The listing builds one solid part. Answer for the finished solid, in the listing's coordinates (mm). Face numbers are marked on the shaded views. A direction names the side the tool comes from. Coordinates: 2 decimals unless noted, no trailing zeros. Write each loop counter-clockwise with the first axis right and the second up, starting at its lowest first coordinate (ties: lowest second). Pieces come first, ordered by that corner, then holes.
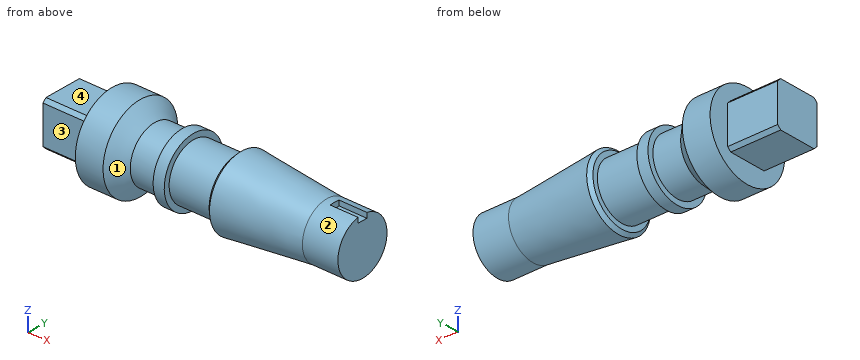
Autodesk Fusion 360 part; units mm, degrees
sketch "Sketch1" plane through (0, 0, 0) normal (0, 1, 0) x (1, 0, 0) in component "Shaft"
  line L0 (0, 0) -> (25, 0)
  line L1 (25, 38) -> (0, 38)
  line L2 (0, 38) -> (0, 0)
  line L3 (25, 38) -> (38, 25)
  line L4 (38, 25) -> (63, 25)
  line L5 (63, 25) -> (63, 30)
  line L6 (63, 30) -> (73, 30)
  line L7 (73, 30) -> (73, 25)
  line L8 (73, 25) -> (113, 25)
  line L9 (113, 25) -> (113, 32.5)
  line L10 (113, 32.5) -> (116, 32.5)
  line L11 (0, 0) -> (193, 0)
  line L12 (116, 32.5) -> (193, 25)
  line L13 (193, 25) -> (225, 25)
  line L14 (225, 25) -> (225, 0)
  line L15 (225, 0) -> (193, 0)
  dimension "d2" = 25
  dimension "d3" = 38
  dimension "d8" = 25
  dimension "d9" = 5
  dimension "d10" = 10
  dimension "d11" = 5
  dimension "d12" = 13
  dimension "d13" = 40
  dimension "d15" = 3
  dimension "d17" = 25
  dimension "d18" = 32
revolve "Revolve1" add sketch "Sketch1" angle 360 about axis through (0, 0, 0) along (1, 0, 0) in component "Shaft"
sketch "Sketch2" plane through (0, 0, 0) normal (-1, 0, 0) x (0, -1, 0) in component "Shaft"
  circle A0 centre (0, 0) radius 38
  line L0 (20, -20) -> (-20, -20)
  line L1 (-20, -20) -> (-20, 20)
  line L2 (-20, 20) -> (20, 20)
  line L3 (20, 20) -> (20, -20)
  line L4 (20, -20) -> (-20, 20) construction
  line L5 (-20, -20) -> (20, 20) construction
  dimension "d20" = 40
  dimension "d21" = 40
extrude "Extrude1" add sketch "Sketch2" along normal blind 45 contours L0 L1 L2 L3 in component "Shaft"
sketch "Sketch3" plane through (225, 0, 0) normal (1, 0, 0) x (0, 1, 0) in component "Shaft"
  circle A0 centre (0, 0) radius 25
  circle A1 centre (0, 0) radius 25
  line L0 (4.5, 20) -> (-4.5, 20)
  arc A2 (4.5, 24.5917) -> (-4.5, 24.5917) centre (0, 0) ccw
  line L1 (4.5, 20) -> (4.5, 24.5917)
  line L2 (-4.5, 20) -> (-4.5, 24.5917)
extrude "Extrude2" cut sketch "Sketch3" against normal blind 25 contours A0 A1 L0 A2 L1 L2 in component "Shaft"
chamfer "Chamfer1" distance 3 angle 45 5 edges at (-22.5, -20, 20) (-22.5, 20, 20) (-22.5, -20, -20) (-22.5, 20, -20) (113, -11.7525, 30.3006) in component "Shaft"
component "Shaft" placed x (1, 0, 0) y (0, 1, 0) z (0, 0, 1) at (0, 0, 0)
1. Section A-A on x = -22 is taken. Give the vertices of the cut face in (y, z).
Results found:
outline: (-20, -17) - (-17, -20) - (17, -20) - (20, -17) - (20, 17) - (17, 20) - (-17, 20) - (-20, 17) - close
2. Find the intervals of material crossed by L1, parallel to X at y = 21, z = 11; L2, parallel to Y at x = 151.5, z = -3; L3, parallel to Z at x = 153.5, y = 3, in increasing order.
Results found:
L1: x = 0 to 225
L2: y = -28.89 to 28.89
L3: z = -28.69 to 28.69
3. A tool of negligible diameter and unlimited length cuts with its end or side. For the marked faces 1, 2, 3 and 4, from which of +Z, -Z, +X, -X, +Y, -Y can it reach the whole face along a straight path? Write none if from no direction.
Results found:
face 1: none
face 2: +X
face 3: +Z, -Z, -X, -Y
face 4: +Z, -X, +Y, -Y
4. Flat-ended cylindrical pins translate along their axes: P1, Ø2.5, axis at x = 218, z = 22.5, coming from the +Y side; P2, Ø17, axis at x = -23, y = 5, coming from the -Z side; P3, Ø5.5, axis at y = -0.5, z = 23, coming from the +X side; P4, Ø8, axis at y = -10, z = 23.5, coming from the -X side. Find the tip coordinate at first contact, or state that the pin passes through.
Results found:
P1: stops at y = 13.17
P2: stops at z = -20
P3: stops at x = 200
P4: stops at x = -45
5. Section D-D on x = 15.5 is taken. Give the vertices of the cut face in (y, z).
Results found:
outline: circle Ø76 at (0, 0)
